The model under review builds one solid part; all positions refer to its coordinate system, in mm. Coordinates: 2 decimals unless noted, no trailing zeros. Write each loop counter-clockwise with the first axis right and the second up, starting at its lowest first coordinate (ties: lowest second). Pieces come first, ordered by that corner, then holes. Notation, with made-up numbers: (-16, 64) -> (28, 64) arc R27 ccw to (28, 94) -> close; hole circle Ø10 at (50, -31). An arc over 180 degrees is marked (long way). Write each question's results on one line, items separated by ' | '.
```python
from build123d import *

# Parameters (mm, degrees)
SKETCH1_W           = 215
SKETCH1_H           = 110
BOSS_EXTRUDE1_DEPTH = 3.175
SKETCH2_W           = 147
SKETCH2_H           = 37
CUT_EXTRUDE1_DEPTH  = 121.79458028
SKETCH3_W           = 15.6
SKETCH3_H           = 50.5
CUT_EXTRUDE2_DEPTH  = 121.79458028
SKETCH5_R           = 1.6
CUT_EXTRUDE4_DEPTH  = 121.79458028
SKETCH6_R           = 1.6
CUT_EXTRUDE5_DEPTH  = 121.79458028
FILLET1_R           = 3
CUT_EXTRUDE6_DEPTH  = 121.79458028


with BuildPart() as part:
    # Sketch1 → Boss-Extrude1 (new body)
    with BuildSketch(Plane(origin=(0, 0, 0), x_dir=(1, 0, 0), z_dir=(0, 1, 0))):
        Rectangle(SKETCH1_W, SKETCH1_H)
    extrude(amount=BOSS_EXTRUDE1_DEPTH)

    # Sketch2 → Cut-Extrude1 (cut, through all)
    with BuildSketch(Plane.XZ):
        Rectangle(SKETCH2_W, SKETCH2_H)
    extrude(amount=-CUT_EXTRUDE1_DEPTH, mode=Mode.SUBTRACT)

    # Sketch3 → Cut-Extrude2 (cut, through all)
    with BuildSketch(Plane.XZ):
        with Locations((-99.7, 0)):
            Rectangle(SKETCH3_W, SKETCH3_H)
    extrude(amount=-CUT_EXTRUDE2_DEPTH, mode=Mode.SUBTRACT)

    # Sketch5 → Cut-Extrude4 (cut, through all)
    with BuildSketch(Plane.XZ):
        with Locations(Location((-79.375, 23.1, 0), (0, 0, 270))):
            Circle(SKETCH5_R)
        with Locations(Location((-79.375, -23.1, 0), (0, 0, 90))):
            Circle(SKETCH5_R)
        with Locations(Location((79.375, -23.1, 0), (0, 0, 270))):
            Circle(SKETCH5_R)
        with Locations(Location((79.375, 23.1, 0), (0, 0, 90))):
            Circle(SKETCH5_R)
        with Locations(Location((-79.375, 35.4, 0), (0, 0, 270))):
            Circle(SKETCH5_R)
        with Locations(Location((-79.375, -35.4, 0), (0, 0, 90))):
            Circle(SKETCH5_R)
        with Locations(Location((79.375, 35.4, 0), (0, 0, 90))):
            Circle(SKETCH5_R)
        with Locations(Location((79.375, -35.4, 0), (0, 0, 270))):
            Circle(SKETCH5_R)
    extrude(amount=-CUT_EXTRUDE4_DEPTH, mode=Mode.SUBTRACT)

    # Sketch6 → Cut-Extrude5 (cut, through all)
    with BuildSketch(Plane(origin=(0, 3.175, 0), x_dir=(1, 0, 0), z_dir=(0, 1, 0))):
        with Locations(Location((37.528255169, 42.068885296, 0), (0, 0, 270))):
            Circle(SKETCH6_R)
        with Locations(Location((0, 42.068885296, 0), (0, 0, 270))):
            Circle(SKETCH6_R)
        with Locations(Location((-37.528255169, 42.068885296, 0), (0, 0, 270))):
            Circle(SKETCH6_R)
        with Locations(Location((-74.528255169, 42.068885296, 0), (0, 0, 270))):
            Circle(SKETCH6_R)
        with Locations(Location((74.528255169, -42.068885296, 0), (0, 0, 270))):
            Circle(SKETCH6_R)
        with Locations(Location((37.528255169, -42.068885296, 0), (0, 0, 270))):
            Circle(SKETCH6_R)
        with Locations(Location((0, -42.068885296, 0), (0, 0, 270))):
            Circle(SKETCH6_R)
        with Locations(Location((-37.528255169, -42.068885296, 0), (0, 0, 270))):
            Circle(SKETCH6_R)
        with Locations(Location((-74.528255169, -42.068885296, 0), (0, 0, 270))):
            Circle(SKETCH6_R)
        with Locations(Location((74.528255169, 42.068885296, 0), (0, 0, 270))):
            Circle(SKETCH6_R)
    extrude(amount=-CUT_EXTRUDE5_DEPTH, mode=Mode.SUBTRACT)

    # Fillet1
    fillet1_edges = [part.edges().sort_by_distance(p)[0] for p in [
        (-73.5, 1.5875, -18.5),
        (-73.5, 1.5875, 18.5),
        (73.5, 1.5875, 18.5),
        (73.5, 1.5875, -18.5),
        (-107.5, 1.5875, -25.25),
        (-107.5, 1.5875, 25.25),
        (-91.9, 1.5875, 25.25),
        (-91.9, 1.5875, -25.25),
        (-107.5, 1.5875, -55),
        (107.5, 1.5875, -55),
        (107.5, 1.5875, 55),
        (-107.5, 1.5875, 55),
    ]]
    fillet(fillet1_edges, radius=FILLET1_R)

    # Sketch7 → Cut-Extrude6 (cut, through all)
    with BuildSketch(Plane.XZ):
        Polygon((-87.4, -46.725), (-88.5, -46.725), (-101.5, -46.725), (-102.6, -46.725), (-102.6, -50.1), (-101.5, -50.1), (-88.5, -50.1), (-87.4, -50.1), align=None)
        Polygon((-101.5, -33.55), (-102.6, -33.55), (-102.6, -36.925), (-101.5, -36.925), (-88.5, -36.925), (-87.4, -36.925), (-87.4, -33.55), (-88.5, -33.55), align=None)
        Polygon((-87.4, 50.1), (-88.5, 50.1), (-101.5, 50.1), (-102.6, 50.1), (-102.6, 46.725), (-101.5, 46.725), (-88.5, 46.725), (-87.4, 46.725), align=None)
        Polygon((-101.5, 36.925), (-102.6, 36.925), (-102.6, 33.55), (-101.5, 33.55), (-88.5, 33.55), (-87.4, 33.55), (-87.4, 36.925), (-88.5, 36.925), align=None)
    extrude(amount=-CUT_EXTRUDE6_DEPTH, mode=Mode.SUBTRACT)


solid = part.part
```
Q1. For line 1 (X direction, y = 2.2, z = 35.4) (3 decimals); line 2 (Z direction, x = -91.5, y = 0.25) (3 decimals); line 3 (X direction, y = 1.7, z = -15.5), list the stretches that pass through material, from the lowest coordinate up. Write a range as from..to.
Solution:
line 1: -107.5..-102.6, -87.4..-80.975, -77.775..77.775, 80.975..107.5 | line 2: -55..-50.1, -46.725..-36.925, -33.55..33.55, 36.925..46.725, 50.1..55 | line 3: -91.9..-73.5, 73.5..107.5
Q2. Add section A-A (z = -11). Write out the cut boundary in (x, y) (3 decimals), plus the area to 3 significant figures.
Solution:
outline: (-91.9, 0) -> (-73.5, 0) -> (-73.5, 3.175) -> (-91.9, 3.175) -> close; (73.5, 0) -> (107.5, 0) -> (107.5, 3.175) -> (73.5, 3.175) -> close | area: 166 mm²
Q3. Add section C-C (y = 1.85). Count the separate pieces of the cut face and the enclosed holes in it, plus the area to 3 significant figures.
Solution:
separate pieces: 1 | enclosed holes: 23 | area: 17,100 mm²
Q4. Clearance check with flat-ended pins moving along their axes: P1, Ø3, axis at x = 0, z = -42.07, coming from the -Y side; P2, Ø1.5, axis at y = 2, z = 8, coming from the -X side. State where each tip first meets the part, or that it passes through.
Solution:
P1: through | P2: x = -91.9
Q5. Add section B-B (x = -25). Write out the cut boundary in (y, z) (3 decimals).
Solution:
outline: (0, -55) -> (3.175, -55) -> (3.175, -18.5) -> (0, -18.5) -> close; (0, 18.5) -> (3.175, 18.5) -> (3.175, 55) -> (0, 55) -> close
